from build123d import *

# Parameters (mm, degrees)
BOSS_EXTRUDE1_DEPTH     = 37.5
SKETCH4_R               = 3
CUT_EXTRUDE3_DEPTH      = 46.067643604
LPATTERN1_COUNT         = 2
LPATTERN1_PITCH         = 28
MIRROR1_COPY_1_SKETCH_R = 3
MIRROR1_COPY_1_DEPTH    = 46.067643604
MIRROR1_COPY_2_SKETCH_R = 3
MIRROR1_COPY_2_DEPTH    = 46.067643604
CHAMFER1_SIZE           = 1.2
SKETCH2_W               = 8
SKETCH2_H               = 16
CUT_EXTRUDE4_DEPTH      = 46.067643604


with BuildPart() as part:
    # Sketch1 → Boss-Extrude1 (new, symmetric)
    with BuildSketch(Plane.XY):
        with BuildLine():
            Line((1.865475811, 3.15), (24.45, 3.15))
            Line((24.45, 3.15), (24.45, 1.65))
            Line((24.45, 1.65), (1.509966887, 1.65))
            ThreePointArc((1.509966887, 1.65), (1.253893127, 1.683342755), (1.014895777, 1.781147541))
            ThreePointArc((1.014895777, 1.781147541), (-1.507477704, -1.389248347), (1.857930963, 0.866367437))
            Line((1.857930963, 0.866367437), (3.217392644, 1.500294829))
            ThreePointArc((3.217392644, 1.500294829), (-2.492742617, -2.527594557), (1.455481127, 3.237912088))
            ThreePointArc((1.455481127, 3.237912088), (1.655818843, 3.172224997), (1.865475811, 3.15))
        make_face()
    extrude(amount=BOSS_EXTRUDE1_DEPTH, both=True)

    # Sketch4 → Cut-Extrude3 (cut, through all)
    with BuildSketch(Plane.XZ.offset(-1.65)):
        with Locations(Location((15.45, 0, 0), (0, 0, 270))):
            Circle(SKETCH4_R)
    cut_extrude3 = extrude(amount=-CUT_EXTRUDE3_DEPTH, mode=Mode.SUBTRACT)

    # LPattern1: Cut-Extrude3 ×2
    with Locations(*[(0, 0, -i * LPATTERN1_PITCH) for i in range(1, LPATTERN1_COUNT)]):
        add(cut_extrude3, mode=Mode.SUBTRACT)

    # Mirror1 copy 1 sketch → Mirror1 copy 1 (cut, through all)
    with BuildSketch(Plane(origin=(0, 1.65, 28), x_dir=(1, 0, 0), z_dir=(0, -1, 0))):
        with Locations((15.45, 0)):
            Circle(MIRROR1_COPY_1_SKETCH_R)
    extrude(amount=-MIRROR1_COPY_1_DEPTH, mode=Mode.SUBTRACT)

    # Mirror1 copy 2 sketch → Mirror1 copy 2 (cut, through all)
    with BuildSketch(Plane.XZ.offset(-1.65)):
        with Locations((15.45, 0)):
            Circle(MIRROR1_COPY_2_SKETCH_R)
    extrude(amount=-MIRROR1_COPY_2_DEPTH, mode=Mode.SUBTRACT)

    # Chamfer1
    chamfer1_edges = [part.edges().sort_by_distance(p)[0] for p in [
        (15.45, 1.65, 3),
        (15.45, 1.65, -25),
        (12.45, 1.65, 28),
    ]]
    chamfer(chamfer1_edges, length=CHAMFER1_SIZE)

    # Sketch2 → Cut-Extrude4 (cut, symmetric)
    with BuildSketch(Plane.XZ.offset(-1.65)):
        with Locations((0.45, -16)):
            Rectangle(SKETCH2_W, SKETCH2_H)
    cut_extrude4 = extrude(amount=CUT_EXTRUDE4_DEPTH, both=True, mode=Mode.SUBTRACT)

    # Mirror2: Cut-Extrude4 across plane
    add(cut_extrude4.mirror(Plane.XY), mode=Mode.SUBTRACT)


solid = part.part
Could you check a few things on this model? Use its own coordinates, in mm. A direction names the side the tool comes from. Coordinates: 2 decimals unless noted, no trailing zeros. Loops run counter-clockwise (first coordinate to the right, second up) from the corner with the lowest first, then second, coordinate; pieces in that order, holes last.
1. I need wall thicknesses on L1, parallel to Y at x = 0, z = 2; L2, parallel to Z at x = 14.75, y = 2.25. Which ranges of each line are inside material? Lowest first, please.
2. Imagine slicing it at C-C (y = -0.25). Please give me the cut outline in (x, z), and give its area (3 significant figures).
3. Imagine slicing it at B-B (x = 0). Please give me the cut outline in (y, z).
4. We'd pull the mould along Y, two halves only. Please class faces 4 (the face through (17.98, 3, -1.61)), 5 (the face through (2.53, 1.18, 0.11)), 6 (the face through (10, 3.15, 1)): released by +Y, released by -Y, zero draft, split by the parting line, or undercut.
5. Imagine slicing it at A-A (z = 0). Please give me the cut outline in (x, y), and give its area (3 significant figures).
6. For P1, Ø1.2, axis at y = 2.5, z = 15, coming from the -X side; P2, Ø9.5, axis at x = 15.45, z = 28, coming from the +Y side; P3, Ø3.5, axis at x = 0, y = 0, coming from the -Z side; P4, Ø9.5, axis at x = 15.45, z = -28, coming from the -Y side, each with a flat end and sliding along its axis, tell me the tip position at first contact or that it passes through.
7. Imagine slicing it at D-D (x = 15.45). Please give me the cut outline in (y, z), and give its area (3 significant figures).
8. For faces 1 (the face through (18.22, 3, 26.85)), 2 (the face through (2.53, 1.18, 30.84)), 3 (the face through (2.2, 0, 8)), which set-ups out of +Z, -Z, +X, -X, +Y, -Y let a thin tool reach every point of the face, with its end or its side?
Computed values:
1. L1: y = -3.55 to -2.05, 2.05 to 3.55
1. L2: z = -37.5 to -31.53, -24.47 to -3.53, 3.53 to 24.47, 31.53 to 37.5
2. outline: (-3.54, -37.5) - (-2.03, -37.5) - (-2.03, -24) - (-3.54, -24) - close; (-3.54, -8) - (-2.03, -8) - (-2.03, 8) - (-3.54, 8) - close; (-3.54, 24) - (-2.03, 24) - (-2.03, 37.5) - (-3.54, 37.5) - close; (2.03, -37.5) - (3.54, -37.5) - (3.54, -24) - (2.03, -24) - close; (2.03, -8) - (3.54, -8) - (3.54, 8) - (2.03, 8) - close; (2.03, 24) - (3.54, 24) - (3.54, 37.5) - (2.03, 37.5) - close
2. area: 130 mm2
3. outline: (-3.55, -37.5) - (-2.05, -37.5) - (-2.05, -24) - (-3.55, -24) - close; (-3.55, -8) - (-2.05, -8) - (-2.05, 8) - (-3.55, 8) - close; (-3.55, 24) - (-2.05, 24) - (-2.05, 37.5) - (-3.55, 37.5) - close; (2.05, -37.5) - (3.55, -37.5) - (3.55, -24) - (2.05, -24) - close; (2.05, -8) - (3.55, -8) - (3.55, 8) - (2.05, 8) - close; (2.05, 24) - (3.55, 24) - (3.55, 37.5) - (2.05, 37.5) - close
4. face 4: zero draft
4. face 5: undercut
4. face 6: released by +Y
5. outline: (1.01, 1.78) arc R1 ccw to (1.51, 1.65) - (11.25, 1.65) - (12.45, 2.85) - (12.45, 3.15) - (1.87, 3.15) arc R1 cw to (1.46, 3.24) arc R3.55 ccw (long way) to (3.22, 1.5) - (1.86, 0.87) arc R2.05 cw (long way) to start; (18.45, 2.85) - (19.65, 1.65) - (24.45, 1.65) - (24.45, 3.15) - (18.45, 3.15) - close
5. area: 48.0 mm2
6. P1: stops at x = 4.45
6. P2: stops at y = 3.15
6. P3: passes through
6. P4: stops at y = 1.65
7. outline: (1.65, -37.5) - (3.15, -37.5) - (3.15, -31) - (2.85, -31) - (1.65, -32.2) - close; (1.65, -23.8) - (2.85, -25) - (3.15, -25) - (3.15, -3) - (2.85, -3) - (1.65, -4.2) - close; (1.65, 4.2) - (2.85, 3) - (3.15, 3) - (3.15, 25) - (2.85, 25) - (1.65, 23.8) - close; (1.65, 32.2) - (2.85, 31) - (3.15, 31) - (3.15, 37.5) - (1.65, 37.5) - close
7. area: 81.2 mm2
8. face 1: +Y, -Y
8. face 2: +Z, -Z
8. face 3: -X, +Y, -Y
